The model under review builds one solid part; all positions refer to its coordinate system, in mm. A direction names the side the tool comes from. Give positions to 0.01 mm unless a question says otherwise; leave off trailing zeros. Order: outer loops, then holes, each group sorted by start corner. A loop starts at its lowest first (then second) coordinate and runs counter-clockwise, first axis right, second up.
```python
from build123d import *

# Parameters (mm, degrees)
SKETCH2_W                    = 100
SKETCH2_H                    = 75
BASE_FLANGE1_DEPTH           = 2.3
EDGE_FLANGE1_STRIP_W         = 13.2
EDGE_FLANGE1_STRIP_H         = 2.3
EDGE_FLANGE1_STRIP_CUT_DEPTH = 75
EDGE_FLANGE1_DEPTH           = 75
EDGE_FLANGE2_STRIP_W         = 13.2
EDGE_FLANGE2_STRIP_H         = 2.3
EDGE_FLANGE2_STRIP_CUT_DEPTH = 75
EDGE_FLANGE2_DEPTH           = 75
CUT_EXTRUDE1_REACH           = 129.475
SKETCH13_R                   = 1.5
SKETCH13_W                   = 10
SKETCH13_H                   = 64.4
SKETCH14_W                   = 10
SKETCH14_H                   = 5
TAB1_DEPTH                   = 2.3
CUT_EXTRUDE2_REACH           = 129.475
SKETCH17_R                   = 0.5
CUT_EXTRUDE3_REACH           = 129.044
SKETCH18_R                   = 1.5


# Sheet-metal steps are written as plain solids
with BuildPart() as part:
    # Sketch2 → Base-Flange1 (new body)
    with BuildSketch(Plane.XY):
        with Locations((50, 37.5)):
            Rectangle(SKETCH2_W, SKETCH2_H)
    extrude(amount=-BASE_FLANGE1_DEPTH)

    # Edge-Flange1 strip (across the edge) → Edge-Flange1 strip cut (cut)
    with BuildSketch(Plane.XZ.offset(-75)):
        with Locations((-2.3, -1.15)):
            Rectangle(EDGE_FLANGE1_STRIP_W, EDGE_FLANGE1_STRIP_H)
    extrude(amount=EDGE_FLANGE1_STRIP_CUT_DEPTH, mode=Mode.SUBTRACT)

    # Edge-Flange1 section (across the edge) → Edge-Flange1 (add)
    with BuildSketch(Plane.XZ.offset(-75)):
        with BuildLine():
            Line((0, 2), (0, 22.7))
            Line((0, 22.7), (2.3, 22.7))
            Line((2.3, 22.7), (2.3, 2))
            ThreePointArc((2.3, 2), (2.885786438, 0.585786438), (4.3, 0))
            Line((4.3, 0), (4.3, -2.3))
            ThreePointArc((4.3, -2.3), (1.259440841, -1.040559159), (0, 2))
        make_face()
    extrude(amount=EDGE_FLANGE1_DEPTH)

    # Edge-Flange2 strip (across the edge) → Edge-Flange2 strip cut (cut)
    with BuildSketch(Plane(origin=(100, 0, 0), x_dir=(-1, 0, 0), z_dir=(0, 1, 0))):
        with Locations((-2.3, -1.15)):
            Rectangle(EDGE_FLANGE2_STRIP_W, EDGE_FLANGE2_STRIP_H)
    extrude(amount=EDGE_FLANGE2_STRIP_CUT_DEPTH, mode=Mode.SUBTRACT)

    # Edge-Flange2 section (across the edge) → Edge-Flange2 (add)
    with BuildSketch(Plane(origin=(100, 0, 0), x_dir=(-1, 0, 0), z_dir=(0, 1, 0))):
        with BuildLine():
            Line((0, 2), (0, 22.7))
            Line((0, 22.7), (2.3, 22.7))
            Line((2.3, 22.7), (2.3, 2))
            ThreePointArc((2.3, 2), (2.885786438, 0.585786438), (4.3, 0))
            Line((4.3, 0), (4.3, -2.3))
            ThreePointArc((4.3, -2.3), (1.259440841, -1.040559159), (0, 2))
        make_face()
    extrude(amount=EDGE_FLANGE2_DEPTH)

    # Sketch13 → Cut-Extrude1 (cut, up to next)
    with BuildSketch(Plane(origin=(0, 0, -2.3), x_dir=(-1, 0, 0), z_dir=(0, 0, -1)), mode=Mode.PRIVATE) as cut_extrude1_sk1:
        with Locations((-66.4, 68.5)):
            Circle(SKETCH13_R)
    cut_extrude1_tool1 = extrude(cut_extrude1_sk1.sketch, amount=-CUT_EXTRUDE1_REACH, mode=Mode.PRIVATE) & part.part
    # Sketch13 → Cut-Extrude1 (cut, up to next)
    with BuildSketch(Plane(origin=(0, 0, -2.3), x_dir=(-1, 0, 0), z_dir=(0, 0, -1)), mode=Mode.PRIVATE) as cut_extrude1_sk2:
        with Locations((-60, 68.5)):
            Circle(SKETCH13_R)
    cut_extrude1_tool2 = extrude(cut_extrude1_sk2.sketch, amount=-CUT_EXTRUDE1_REACH, mode=Mode.PRIVATE) & part.part
    # Sketch13 → Cut-Extrude1 (cut, up to next)
    with BuildSketch(Plane(origin=(0, 0, -2.3), x_dir=(-1, 0, 0), z_dir=(0, 0, -1)), mode=Mode.PRIVATE) as cut_extrude1_sk3:
        with Locations((-41, 68.5)):
            Circle(SKETCH13_R)
    cut_extrude1_tool3 = extrude(cut_extrude1_sk3.sketch, amount=-CUT_EXTRUDE1_REACH, mode=Mode.PRIVATE) & part.part
    # Sketch13 → Cut-Extrude1 (cut, up to next)
    with BuildSketch(Plane(origin=(0, 0, -2.3), x_dir=(-1, 0, 0), z_dir=(0, 0, -1)), mode=Mode.PRIVATE) as cut_extrude1_sk4:
        with Locations((-33, 68.5)):
            Circle(SKETCH13_R)
    cut_extrude1_tool4 = extrude(cut_extrude1_sk4.sketch, amount=-CUT_EXTRUDE1_REACH, mode=Mode.PRIVATE) & part.part
    # Sketch13 → Cut-Extrude1 (cut, up to next)
    with BuildSketch(Plane(origin=(0, 0, -2.3), x_dir=(-1, 0, 0), z_dir=(0, 0, -1)), mode=Mode.PRIVATE) as cut_extrude1_sk5:
        with Locations((-41, 6.5)):
            Circle(SKETCH13_R)
    cut_extrude1_tool5 = extrude(cut_extrude1_sk5.sketch, amount=-CUT_EXTRUDE1_REACH, mode=Mode.PRIVATE) & part.part
    # Sketch13 → Cut-Extrude1 (cut, up to next)
    with BuildSketch(Plane(origin=(0, 0, -2.3), x_dir=(-1, 0, 0), z_dir=(0, 0, -1)), mode=Mode.PRIVATE) as cut_extrude1_sk6:
        with Locations((-33, 6.5)):
            Circle(SKETCH13_R)
    cut_extrude1_tool6 = extrude(cut_extrude1_sk6.sketch, amount=-CUT_EXTRUDE1_REACH, mode=Mode.PRIVATE) & part.part
    # Sketch13 → Cut-Extrude1 (cut, up to next)
    with BuildSketch(Plane(origin=(0, 0, -2.3), x_dir=(-1, 0, 0), z_dir=(0, 0, -1)), mode=Mode.PRIVATE) as cut_extrude1_sk7:
        Polygon((-77, 0), (-53, 0), (-53, 10), (-43, 10), (-43, 15), (-53, 15), (-53, 60), (-77, 60), align=None)
    cut_extrude1_tool7 = extrude(cut_extrude1_sk7.sketch, amount=-CUT_EXTRUDE1_REACH, mode=Mode.PRIVATE) & part.part
    # Sketch13 → Cut-Extrude1 (cut, up to next)
    with BuildSketch(Plane(origin=(0, 0, -2.3), x_dir=(-1, 0, 0), z_dir=(0, 0, -1)), mode=Mode.PRIVATE) as cut_extrude1_sk8:
        with Locations((-87.5, 37.5)):
            Rectangle(SKETCH13_W, SKETCH13_H)
    cut_extrude1_tool8 = extrude(cut_extrude1_sk8.sketch, amount=-CUT_EXTRUDE1_REACH, mode=Mode.PRIVATE) & part.part
    # Sketch13 → Cut-Extrude1 (cut, up to next)
    with BuildSketch(Plane(origin=(0, 0, -2.3), x_dir=(-1, 0, 0), z_dir=(0, 0, -1)), mode=Mode.PRIVATE) as cut_extrude1_sk9:
        with Locations((-12.5, 37.5)):
            Rectangle(SKETCH13_W, SKETCH13_H)
    cut_extrude1_tool9 = extrude(cut_extrude1_sk9.sketch, amount=-CUT_EXTRUDE1_REACH, mode=Mode.PRIVATE) & part.part
    add(cut_extrude1_tool1.solids().sort_by_distance((66.4, 68.5, -2.3))[0], mode=Mode.SUBTRACT)
    add(cut_extrude1_tool2.solids().sort_by_distance((60, 68.5, -2.3))[0], mode=Mode.SUBTRACT)
    add(cut_extrude1_tool3.solids().sort_by_distance((41, 68.5, -2.3))[0], mode=Mode.SUBTRACT)
    add(cut_extrude1_tool4.solids().sort_by_distance((33, 68.5, -2.3))[0], mode=Mode.SUBTRACT)
    add(cut_extrude1_tool5.solids().sort_by_distance((41, 6.5, -2.3))[0], mode=Mode.SUBTRACT)
    add(cut_extrude1_tool6.solids().sort_by_distance((33, 6.5, -2.3))[0], mode=Mode.SUBTRACT)
    add(cut_extrude1_tool7.solids().sort_by_distance((64.42953, 29.412752, -2.3))[0], mode=Mode.SUBTRACT)
    add(cut_extrude1_tool8.solids().sort_by_distance((87.5, 37.5, -2.3))[0], mode=Mode.SUBTRACT)
    add(cut_extrude1_tool9.solids().sort_by_distance((12.5, 37.5, -2.3))[0], mode=Mode.SUBTRACT)

    # Sketch14 → Tab1 (add)
    with BuildSketch(Plane(origin=(0, 0, -2.3), x_dir=(-1, 0, 0), z_dir=(0, 0, -1))):
        with Locations((-87.5, 37.5)):
            Rectangle(SKETCH14_W, SKETCH14_H)
        with Locations((-12.5, 37.5)):
            Rectangle(SKETCH14_W, SKETCH14_H)
    extrude(amount=-TAB1_DEPTH)

    # Sketch17 → Cut-Extrude2 (cut, up to next)
    with BuildSketch(Plane(origin=(0, 0, -2.3), x_dir=(-1, 0, 0), z_dir=(0, 0, -1)), mode=Mode.PRIVATE) as cut_extrude2_sk1:
        with Locations((-94.1, 56.5)):
            Circle(SKETCH17_R)
    cut_extrude2_tool1 = extrude(cut_extrude2_sk1.sketch, amount=-CUT_EXTRUDE2_REACH, mode=Mode.PRIVATE) & part.part
    # Sketch17 → Cut-Extrude2 (cut, up to next)
    with BuildSketch(Plane(origin=(0, 0, -2.3), x_dir=(-1, 0, 0), z_dir=(0, 0, -1)), mode=Mode.PRIVATE) as cut_extrude2_sk2:
        with Locations((-94.1, 19.5)):
            Circle(SKETCH17_R)
    cut_extrude2_tool2 = extrude(cut_extrude2_sk2.sketch, amount=-CUT_EXTRUDE2_REACH, mode=Mode.PRIVATE) & part.part
    # Sketch17 → Cut-Extrude2 (cut, up to next)
    with BuildSketch(Plane(origin=(0, 0, -2.3), x_dir=(-1, 0, 0), z_dir=(0, 0, -1)), mode=Mode.PRIVATE) as cut_extrude2_sk3:
        with Locations((-80.9, 19.5)):
            Circle(SKETCH17_R)
    cut_extrude2_tool3 = extrude(cut_extrude2_sk3.sketch, amount=-CUT_EXTRUDE2_REACH, mode=Mode.PRIVATE) & part.part
    # Sketch17 → Cut-Extrude2 (cut, up to next)
    with BuildSketch(Plane(origin=(0, 0, -2.3), x_dir=(-1, 0, 0), z_dir=(0, 0, -1)), mode=Mode.PRIVATE) as cut_extrude2_sk4:
        with Locations((-80.9, 56.5)):
            Circle(SKETCH17_R)
    cut_extrude2_tool4 = extrude(cut_extrude2_sk4.sketch, amount=-CUT_EXTRUDE2_REACH, mode=Mode.PRIVATE) & part.part
    # Sketch17 → Cut-Extrude2 (cut, up to next)
    with BuildSketch(Plane(origin=(0, 0, -2.3), x_dir=(-1, 0, 0), z_dir=(0, 0, -1)), mode=Mode.PRIVATE) as cut_extrude2_sk5:
        with Locations((-19.1, 19.5)):
            Circle(SKETCH17_R)
    cut_extrude2_tool5 = extrude(cut_extrude2_sk5.sketch, amount=-CUT_EXTRUDE2_REACH, mode=Mode.PRIVATE) & part.part
    # Sketch17 → Cut-Extrude2 (cut, up to next)
    with BuildSketch(Plane(origin=(0, 0, -2.3), x_dir=(-1, 0, 0), z_dir=(0, 0, -1)), mode=Mode.PRIVATE) as cut_extrude2_sk6:
        with Locations((-5.9, 19.5)):
            Circle(SKETCH17_R)
    cut_extrude2_tool6 = extrude(cut_extrude2_sk6.sketch, amount=-CUT_EXTRUDE2_REACH, mode=Mode.PRIVATE) & part.part
    # Sketch17 → Cut-Extrude2 (cut, up to next)
    with BuildSketch(Plane(origin=(0, 0, -2.3), x_dir=(-1, 0, 0), z_dir=(0, 0, -1)), mode=Mode.PRIVATE) as cut_extrude2_sk7:
        with Locations((-5.9, 56.5)):
            Circle(SKETCH17_R)
    cut_extrude2_tool7 = extrude(cut_extrude2_sk7.sketch, amount=-CUT_EXTRUDE2_REACH, mode=Mode.PRIVATE) & part.part
    # Sketch17 → Cut-Extrude2 (cut, up to next)
    with BuildSketch(Plane(origin=(0, 0, -2.3), x_dir=(-1, 0, 0), z_dir=(0, 0, -1)), mode=Mode.PRIVATE) as cut_extrude2_sk8:
        with Locations((-19.1, 56.5)):
            Circle(SKETCH17_R)
    cut_extrude2_tool8 = extrude(cut_extrude2_sk8.sketch, amount=-CUT_EXTRUDE2_REACH, mode=Mode.PRIVATE) & part.part
    add(cut_extrude2_tool1.solids().sort_by_distance((94.1, 56.5, -2.3))[0], mode=Mode.SUBTRACT)
    add(cut_extrude2_tool2.solids().sort_by_distance((94.1, 19.5, -2.3))[0], mode=Mode.SUBTRACT)
    add(cut_extrude2_tool3.solids().sort_by_distance((80.9, 19.5, -2.3))[0], mode=Mode.SUBTRACT)
    add(cut_extrude2_tool4.solids().sort_by_distance((80.9, 56.5, -2.3))[0], mode=Mode.SUBTRACT)
    add(cut_extrude2_tool5.solids().sort_by_distance((19.1, 19.5, -2.3))[0], mode=Mode.SUBTRACT)
    add(cut_extrude2_tool6.solids().sort_by_distance((5.9, 19.5, -2.3))[0], mode=Mode.SUBTRACT)
    add(cut_extrude2_tool7.solids().sort_by_distance((5.9, 56.5, -2.3))[0], mode=Mode.SUBTRACT)
    add(cut_extrude2_tool8.solids().sort_by_distance((19.1, 56.5, -2.3))[0], mode=Mode.SUBTRACT)

    # Sketch18 → Cut-Extrude3 (cut, up to next)
    with BuildSketch(Plane(origin=(100, 0, 0), x_dir=(0, 0, -1), z_dir=(1, 0, 0)), mode=Mode.PRIVATE) as cut_extrude3_sk1:
        with Locations((-14.7, 14.5)):
            Circle(SKETCH18_R)
    cut_extrude3_tool1 = extrude(cut_extrude3_sk1.sketch, amount=-CUT_EXTRUDE3_REACH, mode=Mode.PRIVATE) & part.part
    add(cut_extrude3_tool1.solids().sort_by_distance((100, 14.5, 14.7))[0], mode=Mode.SUBTRACT)


solid = part.part
```
Item 1: Take a section at B-B (y = 42). Give the boundary of the cut face in (x, z), and give its area (3 significant figures).
Values found:
outline: (0, 2) arc R4.3 ccw to (4.3, -2.3) - (7.5, -2.3) - (7.5, 0) - (4.3, 0) arc R2 cw to (2.3, 2) - (2.3, 22.7) - (0, 22.7) - close; (17.5, -2.3) - (53, -2.3) - (53, 0) - (17.5, 0) - close; (77, -2.3) - (82.5, -2.3) - (82.5, 0) - (77, 0) - close; (92.5, -2.3) - (95.7, -2.3) arc R4.3 ccw to (100, 2) - (100, 22.7) - (97.7, 22.7) - (97.7, 2) arc R2 cw to (95.7, 0) - (92.5, 0) - close
area: 227 mm2
Item 2: For faces 1 (the flat face through (48, 10, -1)), 2 (the flat face through (77, 30, -1)), 3 (the flat face through (49, 38, 0)), list the 3-axis set-ups (+Z, -Z, +X, -X, +Y, -Y) from which the entire face can be reached by the end or side of a thin tool; tool diameter is ignored.
Values found:
face 1: +Z, -Z
face 2: +Z, -Z, -Y
face 3: +Z, +Y, -Y
Item 3: Take a section at A-A (x = 66.4). Give the boundary of the cut face in (y, z).
Values found:
outline: (60, -2.3) - (67, -2.3) - (67, 0) - (60, 0) - close; (70, -2.3) - (75, -2.3) - (75, 0) - (70, 0) - close
Item 4: For line 1 (Y direction, x = 41, z = -1.4); line 2 (Y direction, x = 5.9, z = -0.75); line 3 (X direction, y = 36, z = 14.5), list the stretches that pass through material, from the lowest coordinate up.
Values found:
line 1: y = 0 to 5, 8 to 67, 70 to 75
line 2: y = 0 to 19, 20 to 56, 57 to 75
line 3: x = 0 to 2.3, 97.7 to 100
Item 5: Draft analysis for pull direction X (two halves, no side actions). For faces 4 (the flat face through (99, 37, 22.7)), 5 (the flat face through (13, 5.3, -1)), 6 (the flat face through (100, 37, 12)), state which applies: released by +X, released by -X, zero draft, split by the parting line, or undercut.
Values found:
face 4: zero draft
face 5: undercut
face 6: released by +X
Item 6: Clearance check with flat-ended pins moving along their axes: pin 1 Ø1.2 at (y, z) = (6, -1.5) entering from +X; pin 2 Ø1.2 at (y, z) = (21, -1) entering from -X; pin 3 Ø2.5 at (y, z) = (14.5, -1) entering from +X. State where each tip first meets the part, or that it passes through.
Values found:
pin 1: stops at x = 98.87
pin 2: stops at x = 0.73
pin 3: stops at x = 99.63
Item 7: Take a section at D-D (x = 84.5). Give the boundary of the cut face in (y, z), and give its area (3 significant figures).
Values found:
outline: (0, -2.3) - (5.3, -2.3) - (5.3, 0) - (0, 0) - close; (35, -2.3) - (40, -2.3) - (40, 0) - (35, 0) - close; (69.7, -2.3) - (75, -2.3) - (75, 0) - (69.7, 0) - close
area: 35.9 mm2
Item 8: Take a section at C-C (z = 14.7). Give the boundary of the cut face in (x, y).
Values found:
outline: (0, 0) - (2.3, 0) - (2.3, 75) - (0, 75) - close; (97.7, 0) - (100, 0) - (100, 13) - (97.7, 13) - close; (97.7, 16) - (100, 16) - (100, 75) - (97.7, 75) - close
